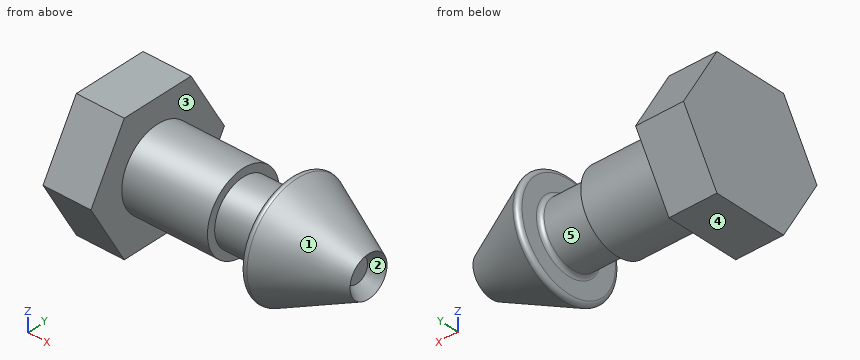
from build123d import *

# Parameters (mm, degrees)
BOSS_EXTRUDE1_DEPTH = 6
FILLET2_R           = 0.5


with BuildPart() as part:
    # Sketch1 → Revolve1 (revolve)
    with BuildSketch(Plane.XY, mode=Mode.PRIVATE) as revolve1_sk:
        Polygon((0, 0), (0, 4.97), (10.72, 4.97), (10.72, 3.97), (16.72, 3.97), (16.72, 7.276374131), (26.39, 2.56), (24.931035164, 1.5), (24.931035164, 0), align=None)
    revolve(revolve1_sk.sketch.rotate(Axis((24.931035164, 0, 0), (-1, 0, 0)), 90), axis=Axis((24.931035164, 0, 0), (-1, 0, 0)))

    # Sketch2 → Boss-Extrude1 (add)
    with BuildSketch(Plane.ZY):
        Polygon((0, 9.237604307), (-8, 4.618802154), (-8, -4.618802154), (0, -9.237604307), (8, -4.618802154), (8, 4.618802154), align=None)
    extrude(amount=BOSS_EXTRUDE1_DEPTH)

    # Fillet2
    fillet2_edges = [part.edges().sort_by_distance(p)[0] for p in [
        (16.72, 0, 7.276374131),
        (16.72, 0, 3.97),
    ]]
    fillet(fillet2_edges, radius=FILLET2_R)


solid = part.part
Check sheet for the modelled part. Datum: model origin and axes. Units: mm. Face numbers are marked on the shaded views. A direction names the side the tool comes from. Round coordinates to 2 decimals unless told otherwise and drop trailing zeros. Order: outer loops, then holes, each group sorted by start corner. A loop starts at its lowest first (then second) coordinate and runs counter-clockwise, first axis right, second up.
(1) Scan lines: probe 1 along X at (y, z) = (-2.75, 7); probe 2 along X at (y, z) = (2, -4.5); probe 3 along X at (y, z) = (0.5, -0.5). Record each from-to range of solid material in increasing order.
(2) Cross-section at B-B, the plane x = -3.5. Enter the section's corners in (y, z).
(3) Cross-section at D-D, the plane y = -8. Enter the section's corners in (x, z).
(4) Draft check along Z on the marked faces 1, 2 and 3. Enter one of: pulls with the +Z half, pulls with the -Z half, needs draft (parallel to the pull), parting line crosses it, or undercut.
(5) Cross-section at C-C, the plane x = 14.5. Enter the section's corners in (y, z), and give its area (3 significant figures).
(6) Access from +Z, -Z, +X, -X, +Y, -Y to the whole of each face (thin tool, end or side, straight path). Record for the marked faces 4 and 5.
(7) Cross-section at A-A, the plane y = 0. Enter the section's corners in (x, z).
(8) Go/stop test with flat-tipped pins: P1, Ø2, axis at x = 6.5, z = -3, coming from the +Y side; P2, Ø3, axis at x = 16.5, z = 2, coming from the +Y side; P3, Ø5, axis at x = 8.5, y = 3, coming from the +Z side. Record where each tip stops, or that it passes through.
Check sheet entries:
1. probe 1: x = -6 to 0
1. probe 2: x = -6 to 10.72, 16.72 to 21.54
1. probe 3: x = -6 to 24.93
2. outline: (-9.24, 0) - (-4.62, -8) - (4.62, -8) - (9.24, 0) - (4.62, 8) - (-4.62, 8) - close
3. outline: (-6, -2.14) - (0, -2.14) - (0, 2.14) - (-6, 2.14) - close
4. face 1: parting line crosses it
4. face 2: undercut
4. face 3: needs draft
5. outline: circle Ø7.94 at (0, 0)
5. area: 49.5 mm2
6. face 4: -Z, +X, -X, +Y, -Y
6. face 5: none
7. outline: (-6, -8) - (0, -8) - (0, -4.97) - (10.72, -4.97) - (10.72, -3.97) - (16.22, -3.97) arc R0.5 cw to (16.72, -4.47) - (16.72, -6.48) arc R0.5 ccw to (17.44, -6.93) - (26.39, -2.56) - (24.93, -1.5) - (24.93, 1.5) - (26.39, 2.56) - (17.44, 6.93) arc R0.5 ccw to (16.72, 6.48) - (16.72, 4.47) arc R0.5 cw to (16.22, 3.97) - (10.72, 3.97) - (10.72, 4.97) - (0, 4.97) - (0, 8) - (-6, 8) - close
8. P1: stops at y = 4.55
8. P2: stops at y = 6.94
8. P3: stops at z = 4.94
